from build123d import *

# Parameters (mm, degrees)
SKETCH5_W                = 33.357089
SKETCH5_H                = 38.1
BOSS_EXTRUDE2_DEPTH      = 1
BOSS_EXTRUDE2_DEPTH_BACK = 78
SKETCH6_W                = 69
SKETCH6_H                = 23.371556831
CUT_EXTRUDE1_DEPTH       = 39.1
SKETCH7_R                = 7.825237577
CUT_EXTRUDE2_DEPTH       = 2
CUT_EXTRUDE2_DEPTH_BACK  = 79
CUT_EXTRUDE3_DEPTH       = 79
SKETCH9_W                = 33
SKETCH9_H                = 38.1
BOSS_EXTRUDE6_DEPTH      = 10
SKETCH11_R               = 7.825237577
CUT_EXTRUDE5_DEPTH       = 79
SKETCH13_W               = 10
SKETCH13_H               = 25.4
CUT_EXTRUDE6_DEPTH       = 11
CUT_EXTRUDE6_DEPTH_BACK  = 7.35
SKETCH14_W               = 11.907690598
SKETCH14_H               = 40
CUT_EXTRUDE8_DEPTH       = 2
CUT_EXTRUDE8_DEPTH_BACK  = 90
SKETCH15_R               = 5.280529318
CUT_EXTRUDE9_DEPTH       = 90
CUT_EXTRUDE9_DEPTH_BACK  = 90
SKETCH16_W               = 38.1
SKETCH16_H               = 16.35
BOSS_EXTRUDE7_DEPTH      = 11


with BuildPart() as part:
    # Sketch5 → Boss-Extrude2 (new body, two sides)
    with BuildSketch(Plane(origin=(0, 0, 0), x_dir=(0, -1, 0), z_dir=(1, 0, 0))) as boss_extrude2_sk:
        with Locations((-10.3285445, 0)):
            Rectangle(SKETCH5_W, SKETCH5_H)
    extrude(amount=BOSS_EXTRUDE2_DEPTH)
    extrude(boss_extrude2_sk.sketch, amount=-BOSS_EXTRUDE2_DEPTH_BACK)

    # Sketch6 → Cut-Extrude1 (cut, through all)
    with BuildSketch(Plane.XY.offset(19.05)):
        with Locations((-33.5, 15.321310585)):
            Rectangle(SKETCH6_W, SKETCH6_H)
    extrude(amount=-CUT_EXTRUDE1_DEPTH, mode=Mode.SUBTRACT)

    # Sketch7 → Cut-Extrude2 (cut, two sides)
    with BuildSketch(Plane(origin=(0, 0, 0), x_dir=(0, 0, -1), z_dir=(1, 0, 0))) as cut_extrude2_sk:
        with Locations((0, 8.496530467)):
            Circle(SKETCH7_R)
    extrude(amount=CUT_EXTRUDE2_DEPTH, mode=Mode.SUBTRACT)
    extrude(cut_extrude2_sk.sketch, amount=-CUT_EXTRUDE2_DEPTH_BACK, mode=Mode.SUBTRACT)

    # Sketch8 → Cut-Extrude3 (cut, through all)
    with BuildSketch(Plane(origin=(0, 0, 0), x_dir=(0, 0, -1), z_dir=(1, 0, 0))):
        with BuildLine():
            Line((-19.05, 3.635532169), (-6.132294733, 3.635532169))
            ThreePointArc((-6.132294733, 3.635532169), (0, 16.321768044), (6.132294733, 3.635532169))
            Line((6.132294733, 3.635532169), (19.05, 3.635532169))
            Line((19.05, 3.635532169), (19.05, 27.007089))
            Line((19.05, 27.007089), (-19.05, 27.007089))
            Line((-19.05, 27.007089), (-19.05, 3.635532169))
        make_face()
        with BuildLine():
            Line((-19.05, 3.635532169), (-6.132294733, 3.635532169))
            ThreePointArc((-6.132294733, 3.635532169), (0, 16.321768044), (6.132294733, 3.635532169))
            Line((6.132294733, 3.635532169), (19.05, 3.635532169))
            Line((19.05, 3.635532169), (19.05, 27.007089))
            Line((19.05, 27.007089), (-19.05, 27.007089))
            Line((-19.05, 27.007089), (-19.05, 3.635532169))
        make_face()
    extrude(amount=-CUT_EXTRUDE3_DEPTH, mode=Mode.SUBTRACT)

    # Sketch9 → Boss-Extrude6 (add)
    with BuildSketch(Plane(origin=(0, 0, 0), x_dir=(1, 0, 0), z_dir=(0, 1, 0))):
        with Locations((-61.5, 0)):
            Rectangle(SKETCH9_W, SKETCH9_H)
    extrude(amount=BOSS_EXTRUDE6_DEPTH)

    # Sketch11 → Cut-Extrude5 (cut, through all)
    with BuildSketch(Plane(origin=(0, 0, 0), x_dir=(0, 0, -1), z_dir=(1, 0, 0))):
        with Locations((0, 8.496530467)):
            Circle(SKETCH11_R)
    extrude(amount=-CUT_EXTRUDE5_DEPTH, mode=Mode.SUBTRACT)

    # Sketch13 → Cut-Extrude6 (cut, two sides)
    with BuildSketch(Plane(origin=(0, 0, 0), x_dir=(1, 0, 0), z_dir=(0, 1, 0))) as cut_extrude6_sk:
        with Locations((-70, -24.7)):
            Rectangle(SKETCH13_W, SKETCH13_H)
        with Locations((-70, 24.7)):
            Rectangle(SKETCH13_W, SKETCH13_H)
    extrude(amount=CUT_EXTRUDE6_DEPTH, mode=Mode.SUBTRACT)
    extrude(cut_extrude6_sk.sketch, amount=-CUT_EXTRUDE6_DEPTH_BACK, mode=Mode.SUBTRACT)

    # Sketch14 → Cut-Extrude8 (cut, two sides)
    with BuildSketch(Plane(origin=(0, 0, 0), x_dir=(0, 0, -1), z_dir=(1, 0, 0))) as cut_extrude8_sk:
        with Locations((0, 20.05843463)):
            Rectangle(SKETCH14_W, SKETCH14_H)
    extrude(amount=CUT_EXTRUDE8_DEPTH, mode=Mode.SUBTRACT)
    extrude(cut_extrude8_sk.sketch, amount=-CUT_EXTRUDE8_DEPTH_BACK, mode=Mode.SUBTRACT)

    # Sketch15 → Cut-Extrude9 (cut, two sides)
    with BuildSketch(Plane(origin=(0, 0, 0), x_dir=(1, 0, 0), z_dir=(0, 1, 0))) as cut_extrude9_sk:
        with Locations((-69.169741906, 0)):
            Circle(SKETCH15_R)
    extrude(amount=CUT_EXTRUDE9_DEPTH, mode=Mode.SUBTRACT)
    extrude(cut_extrude9_sk.sketch, amount=-CUT_EXTRUDE9_DEPTH_BACK, mode=Mode.SUBTRACT)

    # Sketch16 → Boss-Extrude7 (add)
    with BuildSketch(Plane(origin=(-45, 0, 0), x_dir=(0, 0, -1), z_dir=(1, 0, 0))):
        with Locations((0, 1.825)):
            Rectangle(SKETCH16_W, SKETCH16_H)
    extrude(amount=-BOSS_EXTRUDE7_DEPTH)


solid = part.part
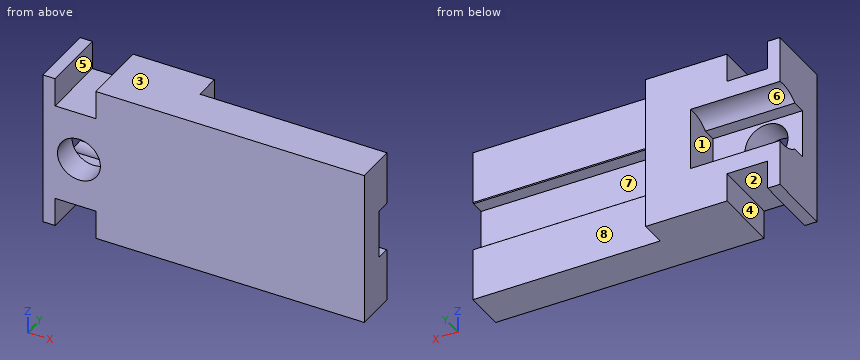
Verification items for the finished model (mm, model axes). Face numbers are marked on the shaded views. A direction names the side the tool comes from. Coordinates: 2 decimals unless noted, no trailing zeros. Order: outer loops, then holes, each group sorted by start corner. A loop starts at its lowest first (then second) coordinate and runs counter-clockwise, first axis right, second up.
1. Sectioned sample at A-A, the plane z = 13. Record the cut outline in (x, y).
Results found:
outline: (-78, -6.35) - (-75, -6.35) - (-75, 10) - (-78, 10) - close; (-65, -6.35) - (1, -6.35) - (1, 3.64) - (-45, 3.64) - (-45, 10) - (-65, 10) - close
2. Sectioned sample at B-B, the plane y = 2.25. Record the cut outline in (x, z).
Results found:
outline: (-78, -19.05) - (-75, -19.05) - (-75, -12) - (-65, -12) - (-65, -19.05) - (1, -19.05) - (1, -5.95) - (-45, -5.95) - (-45, 5.95) - (1, 5.95) - (1, 19.05) - (-65, 19.05) - (-65, 12) - (-75, 12) - (-75, 19.05) - (-78, 19.05) - (-78, 5.95) - (-56, 5.95) - (-56, -5.95) - (-78, -5.95) - close
3. Release check for a two-part mould opening along X. For the marked faces 1, 2 and 3 record: +X half, -X half, draft (parallel to the pull), parting line (faces both ways), or undercut.
Results found:
face 1: -X half
face 2: undercut
face 3: draft
4. Set-up check for the marked faces 4, 5, 6, 7 and 8: record each of +Z, -Z, +X, -X, +Y, -Y from which the full face is reachable in a straight line by a thin tool's end or side.
Results found:
face 4: -Z, +Y, -Y
face 5: +Z, +Y, -Y
face 6: -X
face 7: +X, +Y
face 8: +Z, -Z, +X, +Y
5. Go/stop test with flat-tipped pins: pin 1 Ø3 at (x, y) = (-68.5, 1) entering from +Z; pin 2 Ø4 at (x, z) = (-21.5, 11) entering from +Y; pin 3 Ø9.5 at (x, z) = (-71, -2.5) entering from +Y. Record where each tip stops, or that it passes through.
Results found:
pin 1: stops at z = 12
pin 2: stops at y = 3.64
pin 3: stops at y = 5.55
6. Scan lines: line 1 (X direction, y = -0.5, z = -16); line 2 (Z direction, x = -61, y = 8.75); line 3 (X direction, y = -2.25, z = 0). Record each from-to range of solid material in increasing order.
Results found:
line 1: x = -78 to -75, -65 to 1
line 2: z = -19.05 to -7.82, 7.82 to 19.05
line 3: x = -78 to -74.45, -63.89 to 1
7. Sectioned sample at C-C, the plane x = -18. Record the cut outline in (y, z), and give its area (3 significant figures).
Results found:
outline: (-6.35, -19.05) - (3.64, -19.05) - (3.64, -6.13) arc R7.83 cw to (3.42, -5.95) - (0.06, -5.95) - (0.06, 5.95) - (3.42, 5.95) arc R7.83 cw to (3.64, 6.13) - (3.64, 19.05) - (-6.35, 19.05) - close
area: 338 mm2
8. Sectioned sample at D-D, the plane y = -1.5. Record the cut outline in (x, z).
Results found:
outline: (-78, -19.05) - (-75, -19.05) - (-75, -12) - (-65, -12) - (-65, -19.05) - (1, -19.05) - (1, 19.05) - (-65, 19.05) - (-65, 12) - (-75, 12) - (-75, 19.05) - (-78, 19.05) - close; hole circle Ø10.56 at (-69.17, 0)
